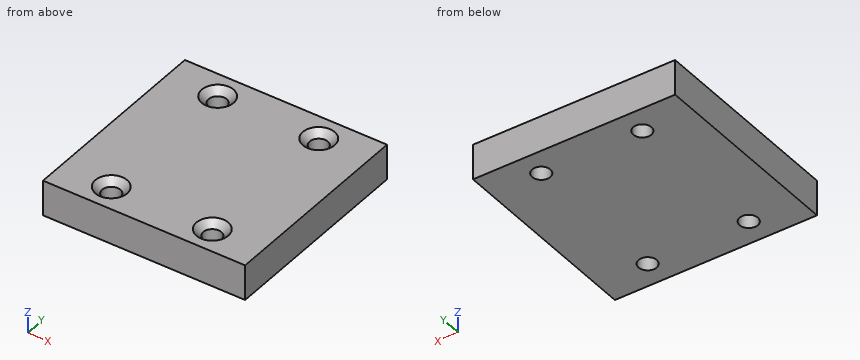
from build123d import *

# Parameters (mm, degrees)
SCHIZZO1_W                   = 40
SCHIZZO1_H                   = 40
ESTRUSIONE_ESTRUSIONE1_DEPTH = 7
RIPETIZIONE_A_L1_COUNT       = 2
RIPETIZIONE_A_L1_PITCH       = 20
RIPETIZIONE_A_L1_COUNT_DIR2  = 2
RIPETIZIONE_A_L1_PITCH_DIR2  = 30


with BuildPart() as part:
    # Schizzo1 → Estrusione-Estrusione1 (new body)
    with BuildSketch(Plane.XY):
        Rectangle(SCHIZZO1_W, SCHIZZO1_H)
    extrude(amount=ESTRUSIONE_ESTRUSIONE1_DEPTH)

    # Schizzo4 → Foro svasato per Vite M3-1 (revolve, cut)
    with BuildSketch(Plane(origin=(-10, 15, 7), x_dir=(0, -1, 0), z_dir=(1, 0, 0))):
        Polygon((0, 0), (0, 11.081549114), (1.8, 10), (1.8, 1.35), (3.15, 0), align=None)
    foro_svasato_per_vite_m3_1 = revolve(axis=Axis((-10, 15, 13.35), (0, 0, -1)), mode=Mode.SUBTRACT)

    # Ripetizione a L1: Foro svasato per Vite M3-1 2 × 2
    with Locations(*[(i * RIPETIZIONE_A_L1_PITCH, -j * RIPETIZIONE_A_L1_PITCH_DIR2, 0) for i in range(RIPETIZIONE_A_L1_COUNT) for j in range(RIPETIZIONE_A_L1_COUNT_DIR2) if (i, j) != (0, 0)]):
        add(foro_svasato_per_vite_m3_1, mode=Mode.SUBTRACT)


solid = part.part
Read the model definition and answer for the solid it produces. Units are mm, in the model's axes. Coordinates: 2 decimals unless noted, no trailing zeros. Write each loop counter-clockwise with the first axis right and the second up, starting at its lowest first coordinate (ties: lowest second). Pieces come first, ordered by that corner, then holes. Notation, with made-up numbers: (16.5, 70.25) -> (48.5, 70.25) arc R26 cw to (48.5, 89.25) -> close; hole circle Ø5 at (6, 70.25). An arc over 180 degrees is marked (long way). Return JSON: item names as keys, results as strings.
(1) This flat-tipped pin is pushed along its axis until it touches: P1, Ø4, axis at x = 10, y = 15, coming from the +Z side. Where does it stop, or does it pass through?
Answers below:
{"P1": "z = 5.85"}
(2) The part is cut by section C-C on y = 15. Give the vertices of the cut face in (x, z).
Answers below:
{"outline": "(-20, 0) -> (-11.8, 0) -> (-11.8, 5.65) -> (-13.15, 7) -> (-20, 7) -> close; (-8.2, 0) -> (8.2, 0) -> (8.2, 5.65) -> (6.85, 7) -> (-6.85, 7) -> (-8.2, 5.65) -> close; (11.8, 0) -> (20, 0) -> (20, 7) -> (13.15, 7) -> (11.8, 5.65) -> close"}
(3) The part is cut by section A-A on x = -10. Give the vertices of the cut face in (y, z).
Answers below:
{"outline": "(-20, 0) -> (-16.8, 0) -> (-16.8, 5.65) -> (-18.15, 7) -> (-20, 7) -> close; (-13.2, 0) -> (13.2, 0) -> (13.2, 5.65) -> (11.85, 7) -> (-11.85, 7) -> (-13.2, 5.65) -> close; (16.8, 0) -> (20, 0) -> (20, 7) -> (18.15, 7) -> (16.8, 5.65) -> close"}
(4) The part is cut by section B-B on z = 3.5. Give the vertices of the cut face in (x, y), then the cut area to 3 significant figures.
Answers below:
{"outline": "(-20, -20) -> (20, -20) -> (20, 20) -> (-20, 20) -> close; hole circle Ø3.6 at (-10, -15); hole circle Ø3.6 at (-10, 15); hole circle Ø3.6 at (10, -15); hole circle Ø3.6 at (10, 15)", "area": "1,560 mm^2"}
(5) Consider line 1 along Y through (x, z) = (-10, 2.5); line 2 along X through (y, z) = (15, 4.4); line 3 along Y through (x, z) = (8, 6.75). Determine where each line is inside the solid, lowest interval first. Write a range as from..to.
Answers below:
{"line 1": "-20..-16.8, -13.2..13.2, 16.8..20", "line 2": "-20..-11.8, -8.2..8.2, 11.8..20", "line 3": "-20..-17.1, -12.9..12.9, 17.1..20"}
(6) The part is cut by section D-D on z = 6.25. Give the vertices of the cut face in (x, y).
Answers below:
{"outline": "(-20, -20) -> (20, -20) -> (20, 20) -> (-20, 20) -> close; hole circle Ø4.8 at (-10, -15); hole circle Ø4.8 at (-10, 15); hole circle Ø4.8 at (10, -15); hole circle Ø4.8 at (10, 15)"}
